Input: part model. Units: mm. Frame: model coordinates. A direction names the side the tool comes from. Coordinates: 2 decimals unless noted, no trailing zeros. Write each loop counter-clockwise with the first axis right and the second up, starting at its lowest first coordinate (ties: lowest second). Pieces come first, ordered by that corner, then holes.
1) Section query C-C (z = 6.5). Output: boundary loops of the cut face in (x, y), then the cut area to 3 significant figures.
2) Section query D-D (y = 42). Output: boundary loops of the cut face in (x, z), then the cut area to 3 significant figures.
3) Pin query (flat end, axial travel): pin 1 Ø1.8 at (x, z) = (-13.5, 1) entering from +Y; pin 2 Ø9 at (x, z) = (0, 0) entering from +Y; pin 3 Ø2 at (x, z) = (-8.5, 6.5) entering from -Y. Return the tip coordinate at first contact, or that it passes through.
4) Section query A-A (x = 2). Output: boundary loops of the cut face in (y, z), then the cut area to 3 significant figures.
5) Line query: L1, parallel to Y at x = 6, z = 0; L2, parallel to X at y = 81, z = 0; L3, parallel to Y at x = -10.5, z = -1.5. Output: solid intervals per line, ascending.
6) Section query B-B (y = 63). Output: boundary loops of the cut face in (x, z).
7) Set-up query: faces 1 (the cylindrical face through (-3.695, 28.846, 1.532)), 2 (the flat face through (3, 18, -3)), 3 (the flat face through (13, 25, 0)), 4 (the flat face through (-13, 25, 0)), 5 (the cylindrical face through (-2.17, 87.04, 9.76)). Return all of +Z, -Z, +X, -X, +Y, -Y with unobstructed straight access to the full face (end or side cutting, diameter ignored); none if empty.
8) Draft query along Z for faces 6 (the flat face through (11, 58, 0)), 7 (the cylindrical face through (-7, 75, -4)), 8 (the cylindrical face through (-9.139, 34.37, -14.334)). Return one class per face: pulls with the +Z half, pulls with the -Z half, needs draft (parallel to the pull), parting line crosses it, or undercut.
Autodesk Inventor part; units mm, degrees
ref_plane "YZ Plane" through (0, 0, 0) normal (1, 0, 0) x (0, 1, 0)
ref_plane "XZ Plane" through (0, 0, 0) normal (0, 1, 0) x (-1, 0, 0)
ref_plane "XY Plane" through (0, 0, 0) normal (0, 0, 1) x (1, 0, 0)
sketch "Sketch1" plane through (0, 0, 0) normal (0, 1, 0) x (-1, 0, 0)
  circle A0 centre (0, 0) radius 4
  circle A1 centre (0, 0) radius 17
  dimension "d0" = 8
  dimension "d1" = 34
extrude "Extrusion1" add sketch "Sketch1" along normal blind 90
sketch "Sketch3" plane through (0, 90, 0) normal (0, 1, 0) x (1, 0, 0)
  line L0 (11, 24.9102) -> (-11, 24.9102)
  line L1 (-11, 24.9102) -> (-11, -24.9102)
  line L2 (-11, -24.9102) -> (11, -24.9102)
  line L3 (11, -24.9102) -> (11, 24.9102)
  line L4 (11, 24.9102) -> (-11, -24.9102) construction
  line L5 (-11, 24.9102) -> (11, -24.9102) construction
  circle A0 centre (0, 0) radius 17
  circle A1 centre (0, 0) radius 17
  point P0 (11, 12.9615)
  point P1 (11, -12.9615)
  point P2 (-11, -12.9615)
  point P3 (-11, 12.9615)
  dimension "d7" = 22
extrude "Extrusion3" cut sketch "Sketch3" against normal blind 65 contours A0 L3 | L1 A0
sketch "Sketch4" plane through (-11, 90, -12.9615) normal (-1, 0, 0) x (0, 0, 1)
  circle A0 centre (12.9615, -50) radius 4
  circle A1 centre (12.9615, -15) radius 4
  line L0 (0, 0) -> (25.923, 0)
  line L1 (29.9615, -90) -> (-4.0385, -90)
  line L2 (0, -65) -> (25.923, -65)
  line L3 (25.923, 0) -> (25.923, -65)
  line L4 (0, 0) -> (25.923, 0)
  line L5 (0, -65) -> (0, 0)
  line L6 (0, -65) -> (25.923, -65)
  line L7 (25.923, 0) -> (25.923, -65)
  line L8 (12.9615, -65) -> (12.9615, -59.6994)
  point P0 (0.995, 0)
  point P1 (15.5881, 0)
  dimension "d12" = 15
  dimension "d15" = 8
  dimension "d17" = 15
extrude "Extrusion4" cut sketch "Sketch4" against normal through all contours A0 | A1
sketch "Sketch5" plane through (0, 0, 0) normal (0, -1, 0) x (1, 0, 0)
  circle A0 centre (0, 0) radius 14.5
  dimension "d18" = 29
extrude "Extrusion5" cut sketch "Sketch5" against normal blind 18
thread "Thread1"
thread "Thread2"
thread "Thread3"
thread "Thread4"
sketch "Sketch6" plane through (0, 90, 0) normal (0, 1, 0) x (1, 0, 0)
  circle A0 centre (0, 0) radius 10
  dimension "d29" = 20
extrude "Extrusion6" cut sketch "Sketch6" against normal blind 6
equation "\"d12\" = d11"
properties part number "Drum" material "Aluminum 6061"
Answer:
1. outline: (-15.71, 0) - (-12.96, 0) - (-12.96, 18) - (12.96, 18) - (12.96, 0) - (15.71, 0) - (15.71, 25) - (11, 25) - (11, 90) - (7.6, 90) - (7.6, 84) - (-7.6, 84) - (-7.6, 90) - (-11, 90) - (-11, 25) - (-15.71, 25) - close
1. area: 1,660 mm2
2. outline: (-11, -12.96) arc R17 ccw to (11, -12.96) - (11, -3.46) - (2, -3.46) arc R4 cw to (-2, -3.46) - (-11, -3.46) - close; (-11, 3.46) - (-2, 3.46) arc R4 cw to (2, 3.46) - (11, 3.46) - (11, 12.96) arc R17 ccw to (-11, 12.96) - close
2. area: 537 mm2
3. pin 1: stops at y = 25
3. pin 2: stops at y = 84
3. pin 3: stops at y = 18
4. outline: (0, -16.88) - (90, -16.88) - (90, -9.8) - (84, -9.8) - (84, -3.46) - (77, -3.46) arc R4 cw to (73, -3.46) - (42, -3.46) arc R4 cw to (38, -3.46) - (18, -3.46) - (18, -14.36) - (0, -14.36) - close; (0, 14.36) - (18, 14.36) - (18, 3.46) - (38, 3.46) arc R4 cw to (42, 3.46) - (73, 3.46) arc R4 cw to (77, 3.46) - (84, 3.46) - (84, 9.8) - (90, 9.8) - (90, 16.88) - (0, 16.88) - close
4. area: 1,940 mm2
5. L1: y = 18 to 36, 44 to 71, 79 to 84
5. L2: x = -11 to -4, 4 to 11
5. L3: y = 18 to 36.29, 43.71 to 71.29, 78.71 to 90
6. outline: (-11, -12.96) arc R17 ccw to (11, -12.96) - (11, 12.96) arc R17 ccw to (-11, 12.96) - close; hole circle Ø8 at (0, 0)
7. face 1: +Y, -Y
7. face 2: -Y
7. face 3: +Z, -Z, +X, +Y
7. face 4: +Z, -Z, -X, +Y
7. face 5: +Y
8. face 6: needs draft
8. face 7: undercut
8. face 8: parting line crosses it
